```python
from build123d import *

# Parameters (mm, degrees)
FILLET1_R          = 0.2
CUT_EXTRUDE1_DEPTH = 2.5


with BuildPart() as part:
    # Sketch1 → Revolve1 (revolve)
    with BuildSketch(Plane.XY):
        Polygon((-0.9, 0), (-0.9, 3), (-0.322649731, 4), (0, 4), (0, 1.785), (0.8, 1.785), (1.5, 2), (16, 2), (16, 0), align=None)
    revolve(axis=Axis((-0.9, 0, 0), (1, 0, 0)))

    # Fillet1
    fillet1_edges = [part.edges().sort_by_distance(p)[0] for p in [
        (0, -1.785, 0),
    ]]
    fillet(fillet1_edges, radius=FILLET1_R)

    # Sketch2 → Cut-Extrude1 (cut)
    with BuildSketch(Plane.ZY.offset(0.9)):
        Polygon((0, 1.154700538), (-1, 0.577350269), (-1, -0.577350269), (0, -1.154700538), (1, -0.577350269), (1, 0.577350269), align=None)
    extrude(amount=-CUT_EXTRUDE1_DEPTH, mode=Mode.SUBTRACT)

    # Sketch3 → Cut-Revolve1 (revolve, cut)
    with BuildSketch(Plane.XY):
        Polygon((1.6, 0), (1.6, 1), (2.200860619, 0), align=None)
    revolve(axis=Axis((1.6, 0, 0), (1, 0, 0)), mode=Mode.SUBTRACT)


solid = part.part
```
Geometry: final body of the model. Coordinates: model frame, mm. A direction names the side the tool comes from. Round coordinates to 2 decimals unless told otherwise and drop trailing zeros. Write each loop counter-clockwise with the first axis right and the second up, starting at its lowest first coordinate (ties: lowest second). Pieces come first, ordered by that corner, then holes. Notation, with made-up numbers: M -16,-7 L 26,-7 A35 cw 26,30 Z; hole C 31,41 d2. An arc over 180 degrees is marked long. Answer in a Markdown table with one row per item. Add a question column.
(1) Reachability of faces 4 (the face through (0.5, 1.7, 0.54)), 5 (the face through (16, 0, 0)), 6 (the face through (0.33, -0.86, -0.51)) from +Z, -Z, +X, -X, +Y, -Y: full face, straight path, thin tool, end or side. Return the list, or none.
(2) Ray query, L1, parallel to Z at x = 6, y = 0.25; L2, parallel to X at y = -1, z = -2.5; L3, parallel to Z at x = 1, y = 0.75. Return the intervals inside material, ascending.
(3) Draft query along Z for faces 1 (the face through (0, -2, -1)), 2 (the face through (0.33, -0.87, 0.49)), 3 (the face through (9, 0, -2)). Return one class per face: pulls with the +Z half, pulls with the -Z half, needs draft (parallel to the pull), parting line crosses it, or undercut.
(4) Cut plane A-A, the plane x = 4.75. Return the cut outline in (y, z).
(5) Contact query for flat-ended pins moving along their axis: pin 1 (1 mm diameter, centred on x = 7.5, y = 0, fed in from -Z); pin 2 (1.5 mm diameter, centred on x = 5, y = 0, fed in from +Z). Output: stop coordinate, or through.
Established:
| question | item | result |
|---|---|---|
| 1 | face 4 | none |
| 1 | face 5 | +Z, -Z, +X, +Y, -Y |
| 1 | face 6 | -X |
| 2 | L1 | -1.98 to 1.98 |
| 2 | L2 | -0.9 to 0 |
| 2 | L3 | -1.69 to -0.7, 0.7 to 1.69 |
| 3 | face 1 | needs draft |
| 3 | face 2 | undercut |
| 3 | face 3 | parting line crosses it |
| 4 | outline | C 0,0 d4 |
| 5 | pin 1 | z = -2 |
| 5 | pin 2 | z = 2 |
